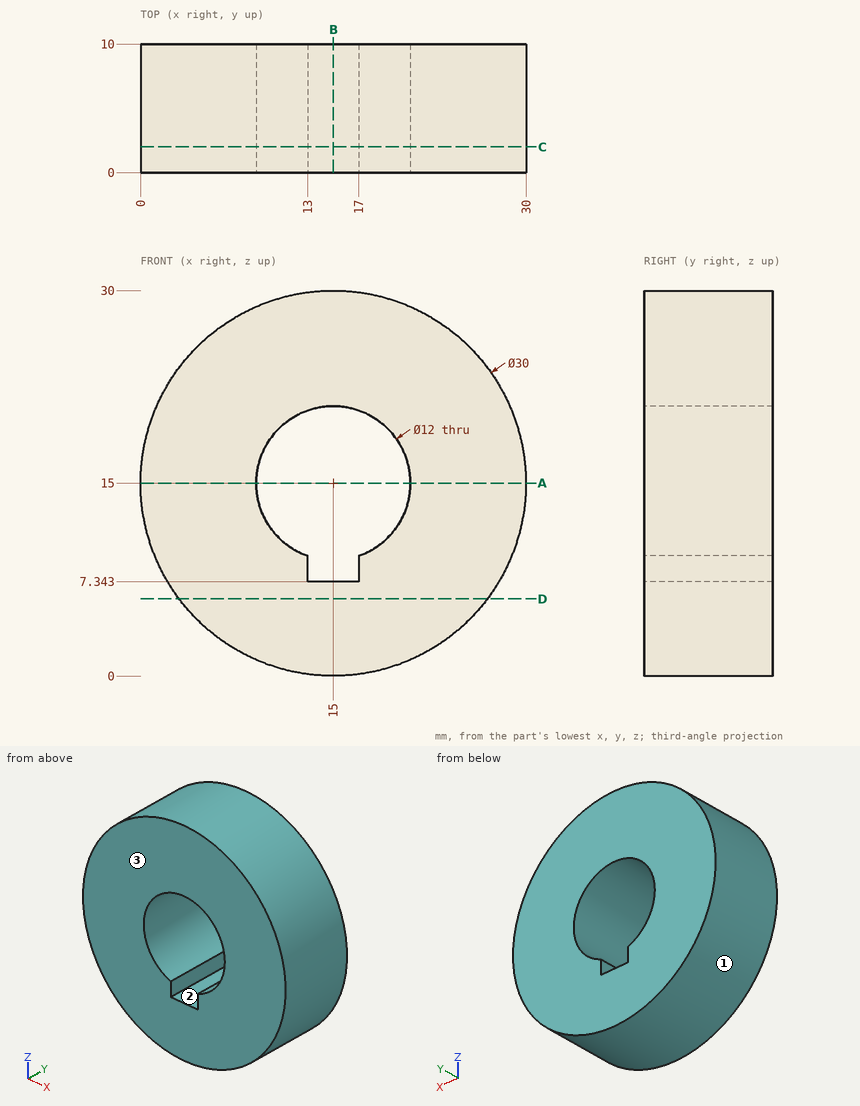
The drawing under review shows one solid part. Ordinate dimensions are in mm from its lowest x, y, z. Coordinates: 2 decimals unless noted, no trailing zeros. Loops run counter-clockwise (first coordinate to the right, second up) from the corner with the lowest first, then second, coordinate; pieces in that order, holes last. Notation, with made-up numbers: (52.25, 61.25) - (86.25, 61.25) arc R30 ccw to (86.25, 89.25) - close; hole circle Ø2 at (24, 20). An arc over 180 degrees is marked (long way). Use CSV: the item, a comma, the result in double quotes. Start each with the question number.
1. Clearance check with flat-ended pins moving along their axes: pin 1 (0.6 mm diameter, centred on y = 6, z = 8.5, fed in from +X); pin 2 (5 mm diameter, centred on y = 5.5, z = 20, fed in from -X); pin 3 (1 mm diameter, centred on y = 7.5, z = 8.5, fed in from -X). State where each tip first meets the part, or that it passes through.
2. Mouldability with a two-part tool opening along Z and no side actions: class the marked faces 1, 2 and 3 as released by +Z, released by -Z, zero draft, split by the parting line, or undercut.
3. Add section B-B on x = 15. Give the boundary of the cut face in (y, z).
4. To check wall thickness, follow probe 1 along X at (y, z) = (3.5, 15); probe 2 along Z at (x, y) = (14.75, 8.75) (1 decimal); probe 3 along X at (y, z) = (1.5, 13.75). State the ranges of each line that lie inside material, in increasing order.
5. Add section D-D on z = 6. Give the boundary of the cut face in (x, y), plus the area to 3 significant figures.
6. Add section C-C on y = 2. Give the boundary of the cut face in (x, z), plus the area to 3 significant figures.
7. Add section A-A on z = 15. Give the boundary of the cut face in (x, y).
Resolved:
1,pin 1,"x = 28.66"
1,pin 2,"x = 0.21"
1,pin 3,"x = 1.25"
2,face 1,"split by the parting line"
2,face 2,"undercut"
2,face 3,"zero draft"
3,outline,"(0, 0) - (10, 0) - (10, 7.34) - (0, 7.34) - close; (0, 21) - (10, 21) - (10, 30) - (0, 30) - close"
4,probe 1,"0 to 9, 21 to 30"
4,probe 2,"0 to 7.3, 21 to 30"
4,probe 3,"0.05 to 9.13, 20.87 to 29.95"
5,outline,"(3, 0) - (27, 0) - (27, 10) - (3, 10) - close"
5,area,"240 mm2"
6,outline,"circle Ø30 at (15, 15); hole (13, 7.34) - (17, 7.34) - (17, 9.34) arc R6 ccw (long way) to (13, 9.34) - close"
6,area,"587 mm2"
7,outline,"(0, 0) - (9, 0) - (9, 10) - (0, 10) - close; (21, 0) - (30, 0) - (30, 10) - (21, 10) - close"
